Part model, mm, in its own coordinate system. Coordinates: 2 decimals unless noted, no trailing zeros. Loops run counter-clockwise (first coordinate to the right, second up) from the corner with the lowest first, then second, coordinate; pieces in that order, holes last. Notation, with made-up numbers: M 71,4.5 L 126,4.5 A31 cw 126,36.5 Z; hole C 50,-16 d5. An arc over 180 degrees is marked long. Answer as a JSON object with one key per item and string values. Group by question number.
1. Drill centre lines: L1, parallel to Y at x = 0, z = 2.6; L2, parallel to X at y = -1, z = 2.1; L3, parallel to Y at x = 305, z = 3.85. Where is each one in solid material? Low to high.
2. Drop flat-ended pins along their axis: pin 1 Ø3 at (x, y) = (-65.5, 3.5) entering from -Z; pin 2 Ø1.3 at (y, z) = (27.5, 1.5) entering from -X; pin 3 Ø1.3 at (y, z) = (-28, 2) entering from +X; pin 4 Ø2 at (x, z) = (102, 2) entering from +Y. Give the stop position or say it passes through.
3. Saw through at A-A on z = 3.5. Count the separate pieces of the cut face and the enclosed holes in it, then the cut area to 3 significant figures.
4. Saw through at B-B on x = 169.5. Write the cut outline in (y, z).
from build123d import *

# Parameters (mm, degrees)
SKETCH1_R           = 2.5
SKETCH1_W           = 4
SKETCH1_H           = 15
BOSS_EXTRUDE1_DEPTH = 4.3


with BuildPart() as part:
    # Sketch1 → Boss-Extrude1 (new body)
    with BuildSketch(Plane.XY):
        Polygon((-340, -25), (-275.1, -25), (-275.1, -29.3), (-204.9, -29.3), (-204.9, -25), (-35.1, -25), (-35.1, -29.3), (35.1, -29.3), (35.1, -25), (204.9, -25), (204.9, -29.3), (275.1, -29.3), (275.1, -25), (340, -25), (340, -7.5), (335.7, -7.5), (335.7, 7.5), (340, 7.5), (340, 25), (275.1, 25), (275.1, 29.3), (204.9, 29.3), (204.9, 25), (35.1, 25), (35.1, 29.3), (-35.1, 29.3), (-35.1, 25), (-204.9, 25), (-204.9, 29.3), (-275.1, 29.3), (-275.1, 25), (-340, 25), (-340, 7.5), (-335.7, 7.5), (-335.7, -7.5), (-340, -7.5), align=None)
        with Locations(Location((0, 0, 0), (0, 0, 180))):
            Circle(SKETCH1_R, mode=Mode.SUBTRACT)
        with Locations((120, 0)):
            Rectangle(SKETCH1_W, SKETCH1_H, mode=Mode.SUBTRACT)
        with Locations((-120, 0)):
            Rectangle(SKETCH1_W, SKETCH1_H, mode=Mode.SUBTRACT)
    extrude(amount=BOSS_EXTRUDE1_DEPTH)


solid = part.part
Outcome:
{
 "1": {"L1": "y = -29.3 to -2.5, 2.5 to 29.3", "L2": "x = -335.7 to -122, -118 to -2.29, 2.29 to 118, 122 to 335.7", "L3": "y = -25 to 25"},
 "2": {"pin 1": "stops at z = 0", "pin 2": "stops at x = -275.1", "pin 3": "stops at x = 275.1", "pin 4": "stops at y = 25"},
 "3": {"separate pieces": "1", "enclosed holes": "3", "area": "35,500 mm²"},
 "4": {"outline": "M -25,0 L 25,0 L 25,4.3 L -25,4.3 Z"}
}
